```python
from build123d import *

# Parameters (mm, degrees)
BOSS_EXTRUDE1_DEPTH = 10
CHAMFER1_SIZE       = 1.5
SKETCH2_W           = 61.34
SKETCH2_H           = 3.8
CUT_EXTRUDE1_DEPTH  = 7


with BuildPart() as part:
    # Sketch1 → Boss-Extrude1 (new body)
    with BuildSketch(Plane(origin=(0, 0, 0), x_dir=(1, 0, 0), z_dir=(0, 1, 0))):
        Polygon((-35.07, 4.5), (-33.57, 6), (33.57, 6), (35.07, 4.5), (35.07, -4.5), (33.57, -6), (-33.57, -6), (-35.07, -4.5), align=None)
    extrude(amount=BOSS_EXTRUDE1_DEPTH)

    # Chamfer1
    chamfer1_edges = [part.edges().sort_by_distance(p)[0] for p in [
        (0, 10, 6),
        (34.32, 10, 5.25),
        (35.07, 10, 0),
        (34.32, 10, -5.25),
        (0, 10, -6),
        (-34.32, 10, -5.25),
        (-35.07, 10, 0),
        (-34.32, 10, 5.25),
    ]]
    chamfer(chamfer1_edges, length=CHAMFER1_SIZE)

    # Sketch2 → Cut-Extrude1 (cut)
    with BuildSketch(Plane.XZ):
        with Locations((0, -1.1)):
            Rectangle(SKETCH2_W, SKETCH2_H)
    extrude(amount=-CUT_EXTRUDE1_DEPTH, mode=Mode.SUBTRACT)


solid = part.part
```
The model under review builds one solid part; all positions refer to its coordinate system, in mm. A direction names the side the tool comes from. Round coordinates to 2 decimals unless told otherwise and drop trailing zeros. Order: outer loops, then holes, each group sorted by start corner. A loop starts at its lowest first (then second) coordinate and runs counter-clockwise, first axis right, second up.
Item 1: Add section A-A, the plane y = 4. State the section outline as (x, z) points, and give its area (3 significant figures).
Working result:
outline: (-35.07, -4.5) - (-33.57, -6) - (33.57, -6) - (35.07, -4.5) - (35.07, 4.5) - (33.57, 6) - (-33.57, 6) - (-35.07, 4.5) - close; hole (-30.67, -3) - (30.67, -3) - (30.67, 0.8) - (-30.67, 0.8) - close
area: 604 mm2
Item 2: Machinability: for faces 1 (the flat face through (0, 7, -1)), 2 (the flat face through (-35.07, 4, 0)), which of the approach directions +Z, -Z, +X, -X, +Y, -Y give a long, thin tool a straight path to every point of the face, cutting with its end or side? Answer none if there is none.
Working result:
face 1: -Y
face 2: +Z, -Z, -X, +Y, -Y
Item 3: To check wall thickness, follow probe 1 along Z at (x, y) = (-1.5, 1.25); probe 2 along X at (y, z) = (5.5, 0.5); probe 3 along Y at (x, z) = (-9.5, -2.5). State the ranges of each line that lie inside material, in increasing order.
Working result:
probe 1: z = -6 to -3, 0.8 to 6
probe 2: x = -35.07 to -30.67, 30.67 to 35.07
probe 3: y = 7 to 10
Item 4: Add section B-B, the plane x = 27. State the section outline as (y, z) points, and give its area (4 significant figures).
Working result:
outline: (0, -6) - (8.5, -6) - (10, -4.5) - (10, 4.5) - (8.5, 6) - (0, 6) - (0, 0.8) - (7, 0.8) - (7, -3) - (0, -3) - close
area: 91.15 mm2
Item 5: Add section D-D, the plane y = 9.25. State the section outline as (x, z) points.
Working result:
outline: (-34.32, -4.19) - (-33.26, -5.25) - (33.26, -5.25) - (34.32, -4.19) - (34.32, 4.19) - (33.26, 5.25) - (-33.26, 5.25) - (-34.32, 4.19) - close
Item 6: Add section C-C, the plane z = -0.5. State the section outline as (x, y) points.
Working result:
outline: (-35.07, 0) - (-30.67, 0) - (-30.67, 7) - (30.67, 7) - (30.67, 0) - (35.07, 0) - (35.07, 8.5) - (33.57, 10) - (-33.57, 10) - (-35.07, 8.5) - close
Item 7: Draft analysis for pull direction Z (two halves, no side actions). For faces 3 (the flat face through (34.31, 9.26, -0.06)), 4 (the flat face through (-30.67, 3, -1)), 5 (the flat face through (0, 4, -6)), 6 (the flat face through (-33.89, 9.094, 4.841)), state which applies: released by +Z, released by -Z, zero draft, split by the parting line, or undercut.
Working result:
face 3: zero draft
face 4: undercut
face 5: released by -Z
face 6: released by +Z
